Geometry: final body of the model. Coordinates: model frame, mm. A direction names the side the tool comes from. Round coordinates to 2 decimals unless told otherwise and drop trailing zeros. Order: outer loops, then holes, each group sorted by start corner. A loop starts at its lowest first (then second) coordinate and runs counter-clockwise, first axis right, second up. Notation, with made-up numbers: M 36.5,35 L 88.5,35 A24 ccw 88.5,46 Z; hole C 66,22.5 d6. An arc over 180 degrees is marked long. Put each result on its own line as item: value. Start each with the question number.
1) First-contact query: P1, Ø4, axis at x = 54.43, y = 75.5, coming from the +Z side; P2, Ø18, axis at x = 14.5, y = 4.5, coming from the -Z side. Flat tips, straight axial feed; report the tip coordinate or a pass-through.
2) Draft query along Y for faces 1 (the cylindrical face through (20.358, 65.727, 21.127)), 2 (the flat face through (0, 69, 12.5)), 3 (the flat face through (-2, 95, 15)). Return one class per face: pulls with the +Y half, pulls with the -Y half, needs draft (parallel to the pull), parting line crosses it, or undercut.
3) Section C-C, the plane y = -10.5. Return loops of the section in (x, z).
4) Section A-A, the plane y = 87. Return loops of the section in (x, z).
5) Access query for faces 4 (the cylindrical face through (-19.642, 65.727, 21.127)), 5 (the flat face through (0, -20, 10.5)). Directions: +Z, -Z, +X, -X, +Y, -Y. A direction counts if a zero-diameter tool reaches every point of the face in a straight line with its end or side. Return the directions, or none.
6) Section B-B, the plane x = 20. Return loops of the section in (y, z).
7) Material intervals for probe 1 along Y at (x, z) = (20, 24.5); probe 2 along X at (y, z) = (2.5, 9.25); probe 3 along Y at (x, z) = (-22, 22.75), sorted ascending. Write a range as [from, to].
from build123d import *

# Parameters (mm, degrees)
SCHIZZO1_W                   = 232
SCHIZZO1_H                   = 190
ESTRUSIONE_ESTRUSIONE1_DEPTH = 30
SCHIZZO4_W                   = 60
SCHIZZO4_H                   = 10.5
TAGLIO_ESTRUSIONE2_DEPTH     = 191
TAP_DRILL_FOR_M5_TAP1_D      = 4.2
M5_CLEARANCE_HOLE1_D         = 5.5
TAP_DRILL_FOR_M5_TAP3_D      = 4.2
TAP_DRILL_FOR_M5_TAP3_DEPTH  = 30
SKETCH8_W                    = 53
SKETCH8_H                    = 52
CUT_EXTRUDE1_DEPTH           = 2


with BuildPart() as part:
    # Schizzo1 → Estrusione-Estrusione1 (new body)
    with BuildSketch(Plane.XY):
        Rectangle(SCHIZZO1_W, SCHIZZO1_H)
    extrude(amount=ESTRUSIONE_ESTRUSIONE1_DEPTH)

    # Schizzo4 → Taglio-Estrusione2 (cut, through all)
    with BuildSketch(Plane(origin=(0, 95, 0), x_dir=(1, 0, 0), z_dir=(0, 1, 0))):
        with Locations((0, -5.25)):
            Rectangle(SCHIZZO4_W, SCHIZZO4_H)
    extrude(amount=-TAGLIO_ESTRUSIONE2_DEPTH, mode=Mode.SUBTRACT)

    # Tap Drill for M5 Tap1 (through all)
    with Locations(Plane(origin=(0, 0, 0), x_dir=(-1, 0, 0), z_dir=(0, 0, -1))):
        with Locations((-54.428761817, 35.5), (-54.428761817, 75.5), (-107.428761817, 35.5), (-107.428761817, -75.5), (-107.428761817, -35.5), (-54.428761817, -35.5), (-54.428761817, -75.5), (54.428761817, -75.5), (54.428761817, -35.5), (107.428761817, -35.5), (107.428761817, -75.5), (107.428761817, 75.5), (107.428761817, 35.5), (54.428761817, 35.5), (54.428761817, 75.5), (-107.428761817, 75.5)):
            Hole(TAP_DRILL_FOR_M5_TAP1_D / 2)

    # M5 Clearance Hole1 (through all)
    with Locations(Plane.XY.offset(30)):
        with Locations((-20, 87), (20, 87), (20, 63), (-20, 63)):
            Hole(M5_CLEARANCE_HOLE1_D / 2)

    # Tap Drill for M5 Tap3
    with Locations(Plane.XY.offset(30)):
        with Locations((-75.75, 7), (-75.75, -80), (75.75, 7), (75.75, -80), (-75.75, -35.79251315), (75.75, -35.79251315)):
            Hole(TAP_DRILL_FOR_M5_TAP3_D / 2, depth=TAP_DRILL_FOR_M5_TAP3_DEPTH)

    # Sketch8 → Cut-Extrude1 (cut)
    with BuildSketch(Plane(origin=(0, 0, 10.5), x_dir=(-1, 0, 0), z_dir=(0, 0, -1))):
        with Locations((0, 69)):
            Rectangle(SKETCH8_W, SKETCH8_H)
    extrude(amount=-CUT_EXTRUDE1_DEPTH, mode=Mode.SUBTRACT)


solid = part.part
Result sheet:
1. P1: passes through
1. P2: stops at z = 10.5
2. face 1: undercut
2. face 2: needs draft
2. face 3: pulls with the +Y half
3. outline: M -116,0 L -30,0 L -30,10.5 L 30,10.5 L 30,0 L 116,0 L 116,30 L -116,30 Z
4. outline: M -116,0 L -30,0 L -30,10.5 L -26.5,10.5 L -26.5,12.5 L -22.75,12.5 L -22.75,30 L -116,30 Z; M -17.25,12.5 L 17.25,12.5 L 17.25,30 L -17.25,30 Z; M 22.75,12.5 L 26.5,12.5 L 26.5,10.5 L 30,10.5 L 30,0 L 116,0 L 116,30 L 22.75,30 Z
5. face 4: +Z, -Z
5. face 5: -Z, +Y, -Y
6. outline: M -95,10.5 L 43,10.5 L 43,12.5 L 60.25,12.5 L 60.25,30 L -95,30 Z; M 65.75,12.5 L 84.25,12.5 L 84.25,30 L 65.75,30 Z; M 89.75,12.5 L 95,12.5 L 95,30 L 89.75,30 Z
7. probe 1: y = [-95, 60.25], [65.75, 84.25], [89.75, 95]
7. probe 2: x = [-116, -30], [30, 116]
7. probe 3: y = [-95, 61.11], [64.89, 85.11], [88.89, 95]
